Autodesk Inventor part; units mm, degrees
ref_plane "YZ Plane" through (0, 0, 0) normal (1, 0, 0) x (0, 1, 0)
ref_plane "XZ Plane" through (0, 0, 0) normal (0, 1, 0) x (-1, 0, 0)
ref_plane "XY Plane" through (0, 0, 0) normal (0, 0, 1) x (1, 0, 0)
sketch "Boceto1" plane through (0, 0, 0) normal (0, 0, 1) x (1, 0, 0)
  line L0 (26.7329, 8.5953) -> (-7.2671, -13.4047) construction
  line L1 (-7.2671, 8.5953) -> (26.7329, -13.4047) construction
  circle A0 centre (9.7329, -2.4047) radius 17.5
  point P0 (0, 0)
  dimension "d13" = 35
extrude "Extrusión1" add sketch "Boceto1" along normal blind 3
sketch "Boceto2" plane through (0, 0, 3) normal (0, 0, 1) x (1, 0, 0)
  line L0 (-7.2671, 8.5953) -> (26.7329, -13.4047) construction
  line L1 (26.7329, 8.5953) -> (-7.2671, -13.4047) construction
  line L2 (-5.0671, 6.3953) -> (24.5329, 6.3953)
  line L3 (24.5329, 6.3953) -> (24.5329, -11.2047)
  line L4 (24.5329, -11.2047) -> (-5.0671, -11.2047)
  line L5 (-5.0671, -11.2047) -> (-5.0671, 6.3953)
  line L6 (-5.0671, 6.3953) -> (24.5329, -11.2047) construction
  line L7 (-5.0671, -11.2047) -> (24.5329, 6.3953) construction
  line L8 (-4.0671, 5.3953) -> (23.5329, 5.3953)
  line L9 (23.5329, 5.3953) -> (23.5329, -10.2047)
  line L10 (23.5329, -10.2047) -> (-4.0671, -10.2047)
  line L11 (-4.0671, -10.2047) -> (-4.0671, 5.3953)
  line L12 (-4.0671, 5.3953) -> (23.5329, -10.2047) construction
  line L13 (23.5329, 5.3953) -> (-4.0671, -10.2047) construction
  point P0 (0, 0)
  point P1 (9.7329, -2.4047)
  dimension "d4" = 29.6
  dimension "d5" = 17.6
  dimension "d6" = 27.6
  dimension "d7" = 15.6
extrude "Extrusión2" add sketch "Boceto2" along normal blind 5
sketch "Boceto5" plane through (9.7329, -2.4047, 0) normal (0, 0, -1) x (-1, 0, 0)
  arc A0 (-13.463, -0.9993) -> (-13.463, 0.9993) centre (0, 0) ccw
  arc A1 (-13.463, 0.9993) -> (-13.463, -0.9993) centre (-13.4997, 0) ccw
  point P0 (9.7329, 2.4047)
  dimension "d14" = 27
  dimension "d15" = 2
hole "Hole1" at (17.4667, -2.2309, 0) direction (0, 0, 1) diameter 2 depth 4
extrude "Extrusión3" cut sketch "Boceto5" against normal blind 0.5
equation "\"Radio_pliegue\" = Grosor"
equation "\"Anchura_desahogo_plegado\" = Grosor"
equation "\"Profundidad_desahogo_plegado\" = 0.5 * Grosor"
equation "\"Tamaño_destalonado\" = 4 * Grosor"
equation "\"Remanente_mínimo\" = 2 * Grosor"
equation "\"Radiodetransición\" = Radio_pliegue"
equation "\"Tamaño_de_radio_de_Jacobi\" = Radio_pliegue"
equation "\"TamañoSeparación\" = Grosor"
properties part number "Tapa2"
The listing builds one solid part. Answer for the finished solid, in the listing's coordinates (mm). A direction names the side the tool comes from. Coordinates: 2 decimals unless noted, no trailing zeros. Order: outer loops, then holes, each group sorted by start corner. A loop starts at its lowest first (then second) coordinate and runs counter-clockwise, first axis right, second up. Notation, with made-up numbers: (-33, 11.5) -> (7, 11.5) arc R13 cw to (7, 20.5) -> close; hole circle Ø5 at (28, 88.25). An arc over 180 degrees is marked (long way). Answer in a Markdown table with one row per item. Add a question column.
Item 1: Determine the mould class of faces 1 (the face through (0.6, 8, 0)), 2 (the face through (24.533, -2, 5)), 3 (the face through (-3.755, -2.984, 0.246)) for opening direction X: +X half, -X half, draft (parallel to the pull), parting line (faces both ways), or undercut.
Item 2: Which of the six approach directions +Z, -Z, +X, -X, +Y, -Y give full straight-line access (tool end or side, diameter ignored) to faces 4 (the face through (10, -10.205, 5)), 5 (the face through (10, -2, 0.5)), 6 (the face through (10, 6.395, 5))?
Item 3: Find section B-B (x = 22.5). Write down the section's boundary in (y, z).
Item 4: Find section D-D (x = -0.5). Write down the section's boundary in (y, z), then the cut area to 3 significant figures.
Item 5: Find section C-C (y = -12.5). Write down the section's boundary in (x, z), then the cut area to 3 significant figures.
Item 6: Find the intervals of material crossed by L1, parallel to Y at x = 16, z = 6.25; L2, parallel to X at y = 3, z = 5.75; L3, parallel to Z at x = 11.5, y = 0.5, in increasing order. Write a range as from..to.
Item 7: Each of these flat-tipped pins is pushed along its axis until it touches: P1, Ø2.5, axis at y = -5, z = 5, coming from the +X side; P2, Ø4, axis at x = 22.5, y = -15.5, coming from the +Z side; P3, Ø3, axis at x = 17.47, y = -2.23, coming from the -Z side. Where does it stop, or does it pass through?
Item 8: Find section A-A (z = 6). Write down the section's boundary in (x, y), then the cut area to 3 significant figures.
Result set:
| question | item | result |
|---|---|---|
| 1 | face 1 | draft |
| 1 | face 2 | +X half |
| 1 | face 3 | undercut |
| 2 | face 4 | +Z |
| 2 | face 5 | -Z |
| 2 | face 6 | +Z, +X, -X, +Y |
| 3 | outline | (-14.37, 0) -> (-6.79, 0) -> (-6.79, 0.5) -> (1.98, 0.5) -> (1.98, 0) -> (9.56, 0) -> (9.56, 3) -> (6.4, 3) -> (6.4, 8) -> (5.4, 8) -> (5.4, 3) -> (-10.2, 3) -> (-10.2, 8) -> (-11.2, 8) -> (-11.2, 3) -> (-14.37, 3) -> close |
| 4 | outline | (-16.6, 0) -> (-11.21, 0) -> (-11.21, 0.5) -> (6.4, 0.5) -> (6.4, 0) -> (11.79, 0) -> (11.79, 3) -> (6.4, 3) -> (6.4, 8) -> (5.4, 8) -> (5.4, 3) -> (-10.2, 3) -> (-10.2, 8) -> (-11.2, 8) -> (-11.2, 3) -> (-16.6, 3) -> close |
| 4 | area | 86.4 mm² |
| 5 | outline | (-4.56, 0) -> (0.77, 0) -> (0.77, 0.5) -> (18.7, 0.5) -> (18.7, 0) -> (24.03, 0) -> (24.03, 3) -> (-4.56, 3) -> close |
| 5 | area | 76.8 mm² |
| 6 | L1 | y = -11.2..-10.2, 5.4..6.4 |
| 6 | L2 | x = -5.07..-4.07, 23.53..24.53 |
| 6 | L3 | z = 0.5..3 |
| 7 | P1 | stops at x = 24.53 |
| 7 | P2 | stops at z = 3 |
| 7 | P3 | stops at z = 0.5 |
| 8 | outline | (-5.07, -11.2) -> (24.53, -11.2) -> (24.53, 6.4) -> (-5.07, 6.4) -> close; hole (-4.07, -10.2) -> (23.53, -10.2) -> (23.53, 5.4) -> (-4.07, 5.4) -> close |
| 8 | area | 90.4 mm² |
